```python
from build123d import *

# Parameters (mm, degrees)
SKETCH1_W           = 60
SKETCH1_H           = 60
BOSS_EXTRUDE1_DEPTH = 10
SKETCH2_W           = 40
SKETCH2_H           = 40
BOSS_EXTRUDE2_DEPTH = 341.83195
FILLET1_R           = 10


with BuildPart() as part:
    # Sketch1 → Boss-Extrude1 (new body)
    with BuildSketch(Plane(origin=(0, 0, 0), x_dir=(1, 0, 0), z_dir=(0, 1, 0))):
        Rectangle(SKETCH1_W, SKETCH1_H)
    extrude(amount=BOSS_EXTRUDE1_DEPTH)

    # Sketch2 → Boss-Extrude2 (add)
    with BuildSketch(Plane(origin=(0, 0, 0), x_dir=(1, 0, 0), z_dir=(0, 1, 0))):
        Rectangle(SKETCH2_W, SKETCH2_H)
    extrude(amount=BOSS_EXTRUDE2_DEPTH)

    # Fillet1
    fillet1_edges = [part.edges().sort_by_distance(p)[0] for p in [
        (20, 175.915975, 20),
        (20, 175.915975, -20),
        (-20, 175.915975, -20),
        (-20, 175.915975, 20),
        (30, 5, 30),
        (-30, 5, 30),
        (-30, 5, -30),
        (30, 5, -30),
    ]]
    fillet(fillet1_edges, radius=FILLET1_R)


solid = part.part
```
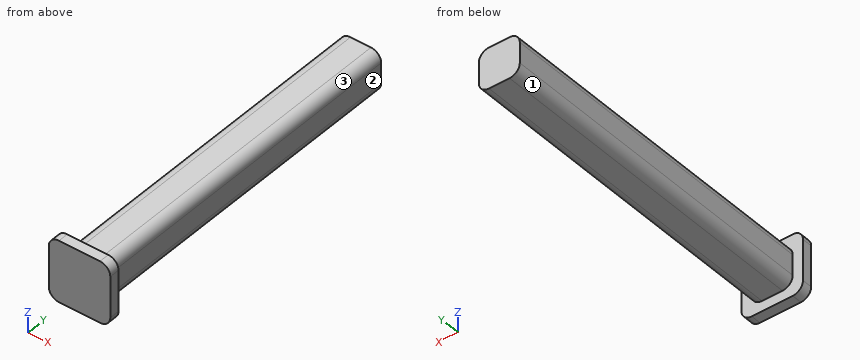
The listing builds one solid part. Answer for the finished solid, in the listing's coordinates (mm). Face numbers are marked on the shaded views. A direction names the side the tool comes from. Round coordinates to 2 decimals unless told otherwise and drop trailing zeros. Loops run counter-clockwise (first coordinate to the right, second up) from the corner with the lowest first, then second, coordinate; pieces in that order, holes last. Notation, with made-up numbers: (-24.5, -30.5) - (-16.5, -30.5) arc R17 ccw to (-16.5, -9.5) - close; hole circle Ø2 at (-3, 28.25). An arc over 180 degrees is marked (long way). Return JSON: item names as keys, results as strings. Group by question number.
1. The part is cut by section A-A on y = 52. Determine the outline of the cut face in (x, z).
2. Each of these flat-tipped pins is pushed along its axis until it touches: P1, Ø16, axis at x = -2, y = 203.5, coming from the -Z side; P2, Ø22, axis at x = -2, y = 162, coming from the +Z side; P3, Ø6, axis at y = 272.5, z = 16, coming from the +X side. Where does it stop, or does it pass through?
3. Consider probe 1 along Y at (x, z) = (-21, -3.5); probe 2 along Z at (x, y) = (-2, 32). Determine where each line is inside the solid, lowest interval first.
4. The part is cut by section B-B on x = 4.5. Determine the outline of the cut face in (y, z).
5. Which of the six approach directions +Z, -Z, +X, -X, +Y, -Y give full straight-line access (tool end or side, diameter ignored) to the marked faces 1, 2 and 3?
6. The part is cut by section C-C on x = -25.5. Determine the outline of the cut face in (y, z), then the cut area to 3 significant figures.
Resolved:
{
 "1": {"outline": "(-20, -10) arc R10 ccw to (-10, -20) - (10, -20) arc R10 ccw to (20, -10) - (20, 10) arc R10 ccw to (10, 20) - (-10, 20) arc R10 ccw to (-20, 10) - close"},
 "2": {"P1": "stops at z = -20", "P2": "stops at z = 20", "P3": "stops at x = 19.54"},
 "3": {"probe 1": "y = 0 to 10", "probe 2": "z = -20 to 20"},
 "4": {"outline": "(0, -30) - (10, -30) - (10, -20) - (341.83, -20) - (341.83, 20) - (10, 20) - (10, 30) - (0, 30) - close"},
 "5": {"face 1": "-Z, -X, +Y", "face 2": "+Z, -Z, +X, +Y", "face 3": "+Z, +X, +Y"},
 "6": {"outline": "(0, -28.35) - (10, -28.35) - (10, 28.35) - (0, 28.35) - close", "area": "567 mm²"}
}
